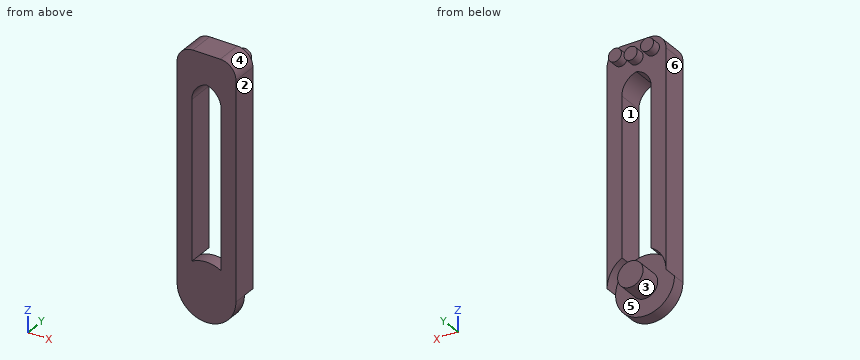
from build123d import *

# Parameters (mm, degrees)
F1_DEPTH    = 1.27
F3_R        = 1.524
F5_T1_DEPTH = 1.27
F2_R        = 1.2397519619
F6_DEPTH    = 2.1971
F4_R        = 0.6356353333
F4_R_2      = 0.6409754112
F7_DEPTH    = 3.429
F9_DEPTH    = 2.54


# Not quite as in the source:
# - a fillet or chamfer that OpenCascade refuses, or shapes differently, is made with other operations: its cross-section is extruded or revolved along the edge and cut away or added


with BuildPart() as f1:
    # F0 (on Front) → F1 (new body)
    with BuildSketch(Plane.XZ):
        with BuildLine():
            ThreePointArc((1.4341250062, 5.3522273875), (2.4839773751, 4.3023750186), (2.8682500124, 2.8682500124))
            Line((2.8682500124, 2.8682500124), (2.8682500124, 25.4276227206))
            Line((2.8682500124, 25.4276227206), (0, 25.4276227206))
            Line((0, 25.4276227206), (-1.4341250062, 25.4276227206))
            Line((-1.4341250062, 25.4276227206), (-2.8682500124, 25.4276227206))
            Line((-2.8682500124, 25.4276227206), (-2.8682500124, 2.8682500124))
            ThreePointArc((-2.8682500124, 2.8682500124), (-2.4839773751, 4.3023750186), (-1.4341250062, 5.3522273875))
            Line((-1.4341250062, 5.3522273875), (-1.4341250062, 22.6080268621))
            Line((-1.4341250062, 22.6080268621), (1.4341250062, 22.6080268621))
            Line((1.4341250062, 22.6080268621), (1.4341250062, 5.3522273875))
        make_face()
        with BuildLine():
            ThreePointArc((-2.8682500124, 2.8682500124), (0, 0), (2.8682500124, 2.8682500124))
            ThreePointArc((2.8682500124, 2.8682500124), (2.4839773751, 4.3023750186), (1.4341250062, 5.3522273875))
            ThreePointArc((1.4341250062, 5.3522273875), (0, 5.7365000248), (-1.4341250062, 5.3522273875))
            ThreePointArc((-1.4341250062, 5.3522273875), (-2.4839773751, 4.3023750186), (-2.8682500124, 2.8682500124))
        make_face()
    extrude(amount=F1_DEPTH)

    # F3
    f3_edges = [f1.edges().sort_by_distance(p)[0] for p in [
        (2.86825, -0.635, 25.427623),
        (-2.86825, -0.635, 25.427623),
    ]]
    fillet(f3_edges, radius=F3_R)

    # F5: fillet of radius 1.905 on 2 edges, made by hand

    # F5_s2 → F5_t1 (join)
    with BuildSketch(Plane.XZ):
        with BuildLine():
            ThreePointArc((-0.4708749938, 22.6080268621), (0.8761634244, 22.0500652803), (1.4341250062, 20.7030268621))
            Line((1.4341250062, 20.7030268621), (1.4341250062, 22.6080268621))
            Line((1.4341250062, 22.6080268621), (-0.4708749938, 22.6080268621))
        make_face()
        with BuildLine():
            ThreePointArc((-1.4341250062, 20.7030268621), (-0.8761634244, 22.0500652803), (0.4708749938, 22.6080268621))
            Line((0.4708749938, 22.6080268621), (-1.4341250062, 22.6080268621))
            Line((-1.4341250062, 22.6080268621), (-1.4341250062, 20.7030268621))
        make_face()
    extrude(amount=F5_T1_DEPTH)

    # F2 (on face) → F6 (join)
    with BuildSketch(Plane(origin=(0, 0, 0), x_dir=(-1, 0, 0), z_dir=(0, 1, 0))):
        with Locations((0, 2.8682500124)):
            Circle(F2_R)
    extrude(amount=F6_DEPTH)

    # F4 (on face) → F7 (join)
    with BuildSketch(Plane.XZ.offset(1.27)):
        with Locations((-1.5970880988, 24.1730304042)):
            Circle(F4_R)
        with Locations((1.5335635452, 24.1730304042)):
            Circle(F4_R)
        with Locations((0, 23.8491314396)):
            Circle(F4_R_2)
    extrude(amount=-F7_DEPTH)

    # F8 (on face) → F9 (join)
    with BuildSketch(Plane.XZ.offset(1.27)):
        with BuildLine():
            ThreePointArc((1.4341250062, 5.3522273875), (2.4839773751, 4.3023750186), (2.8682500124, 2.8682500124))
            Line((2.8682500124, 2.8682500124), (2.8682500124, 23.9036227206))
            ThreePointArc((2.8682500124, 23.9036227206), (1.7143439066, 22.42524303), (0, 23.1855921473))
            ThreePointArc((0, 23.1855921473), (-1.7143439066, 22.42524303), (-2.8682500124, 23.9036227206))
            Line((-2.8682500124, 23.9036227206), (-2.8682500124, 22.548914654))
            Line((-2.8682500124, 22.548914654), (-2.8682500124, 2.8682500124))
            ThreePointArc((-2.8682500124, 2.8682500124), (-2.4839773751, 4.3023750186), (-1.4341250062, 5.3522273875))
            Line((-1.4341250062, 5.3522273875), (-1.4341250062, 20.7030268621))
            ThreePointArc((-1.4341250062, 20.7030268621), (-1.0334590554, 21.8717886293), (0, 22.548914654))
            ThreePointArc((0, 22.548914654), (1.0334590554, 21.8717886293), (1.4341250062, 20.7030268621))
            Line((1.4341250062, 20.7030268621), (1.4341250062, 5.3522273875))
        make_face()
        with BuildLine():
            ThreePointArc((-2.8682500124, 23.9036227206), (-1.7143439066, 22.42524303), (0, 23.1855921473))
            ThreePointArc((0, 23.1855921473), (-0.1797499876, 23.9036227206), (0, 24.6216532939))
            ThreePointArc((0, 24.6216532939), (-0.5605736103, 25.2106909273), (-1.3442500124, 25.4276227206))
            ThreePointArc((-1.3442500124, 25.4276227206), (-2.4218807469, 24.9812534551), (-2.8682500124, 23.9036227206))
        make_face()
        with BuildLine():
            ThreePointArc((0, 23.1855921473), (1.7143439066, 22.42524303), (2.8682500124, 23.9036227206))
            ThreePointArc((2.8682500124, 23.9036227206), (2.4218807469, 24.9812534551), (1.3442500124, 25.4276227206))
            ThreePointArc((1.3442500124, 25.4276227206), (0.5605736103, 25.2106909273), (0, 24.6216532939))
            ThreePointArc((0, 24.6216532939), (0.1341296782, 24.2737166148), (0.1797499876, 23.9036227206))
            ThreePointArc((0.1797499876, 23.9036227206), (0.1341296782, 23.5335288264), (0, 23.1855921473))
        make_face()
        with BuildLine():
            ThreePointArc((0, 24.6216532939), (-0.1797499876, 23.9036227206), (0, 23.1855921473))
            ThreePointArc((0, 23.1855921473), (0.1341296782, 23.5335288264), (0.1797499876, 23.9036227206))
            ThreePointArc((0.1797499876, 23.9036227206), (0.1341296782, 24.2737166148), (0, 24.6216532939))
        make_face()
        with BuildLine():
            ThreePointArc((0, 24.6216532939), (0.5605736103, 25.2106909273), (1.3442500124, 25.4276227206))
            Line((1.3442500124, 25.4276227206), (-1.3442500124, 25.4276227206))
            ThreePointArc((-1.3442500124, 25.4276227206), (-0.5605736103, 25.2106909273), (0, 24.6216532939))
        make_face()
    extrude(amount=-F9_DEPTH)


solid = f1.part
Part model, mm, in its own coordinate system. Face numbers are marked on the shaded views. A direction names the side the tool comes from. Coordinates: 2 decimals unless noted, no trailing zeros. Loops run counter-clockwise (first coordinate to the right, second up) from the corner with the lowest first, then second, coordinate; pieces in that order, holes last. Notation, with made-up numbers: M 8.5,-13.5 L 48.5,-13.5 A29 cw 48.5,6.5 Z; hole C -39,-38 d10. An arc over 180 degrees is marked long. Use a Markdown table: item, result. Add a question column.
Q1. Mould opens along Z. For the marked faces 4, 5 and 6 say: +Z half, -Z half, draft (parallel to the pull), parting line (faces both ways), or undercut.
Q2. Cut at D-D (x = 2.45). Write the cut outline in (y, z), and give its area (3 significant figures).
Q3. Cut at C-C (y = -0.6). Write the cut outline in (x, z) (1 decimal), and give its area (3 significant figures).
Q4. Probe L1, parallel to X at y = 0.9, z = 15; L2, parallel to Z at x = 0, y = 1.4; L3, parallel to Y at x = 2.3, z = 5.25. List the from-to ranges inside material, lowest first.
Q5. Cut at A-A (z = 9). Write the cut outline in (x, y).
Q6. Pin check, flat tips, straight feed: P1, Ø1, axis at x = 1, z = 14, coming from the +Y side; P2, Ø1, axis at x = 1.5, z = 24.5, coming from the +Y side; P3, Ø2, axis at x = -1.5, y = -0.5, coming from the -Z side; P4, Ø1.5, axis at x = 0, z = 15.5, coming from the -Y side. Stop position of each tip, or through.
Q7. Which spindle directions (+Z, -Z, +X, -X, +Y, -Y) get a long thin tool onto all of the face, cutting with end or side? Do the marked faces 1, 2 and 3. Say none if no direction does.
Q8. Cut at B-B (y = 0.65). Write the cut outline in (x, z) (1 decimal).
Worked out:
| question | item | result |
|---|---|---|
| 1 | face 4 | +Z half |
| 1 | face 5 | undercut |
| 1 | face 6 | draft |
| 2 | outline | M -1.27,1.38 L 0,1.38 L 0,4.36 L 1.27,4.36 L 1.27,24.95 L -1.27,24.95 Z |
| 2 | area | 56.1 mm2 |
| 3 | outline | M -2.9,2.9 A2.9 ccw 2.9,2.9 L 2.9,23.9 A1.5 ccw 1.3,25.4 L -1.3,25.4 A1.5 ccw -2.9,23.9 Z; hole M -1.4,5.4 A2.9 cw 1.4,5.4 L 1.4,20.7 A1.9 ccw 0,22.5 A1.9 ccw -1.4,20.7 Z |
| 3 | area | 94.1 mm2 |
| 4 | L1 | x = -2.87 to -1.43, 1.43 to 2.87 |
| 4 | L2 | z = 1.63 to 4.11, 23.21 to 24.49 |
| 4 | L3 | y = -1.27 to 1.27 |
| 5 | outline | M -2.87,-1.27 L -1.43,-1.27 L -1.43,1.27 L -2.87,1.27 Z; M 1.43,-1.27 L 2.87,-1.27 L 2.87,1.27 L 1.43,1.27 Z |
| 6 | P1 | stops at y = 1.27 |
| 6 | P2 | stops at y = 2.16 |
| 6 | P3 | stops at z = 0.04 |
| 6 | P4 | passes through |
| 7 | face 1 | +Y, -Y |
| 7 | face 2 | +Z, -Z, +X, +Y, -Y |
| 7 | face 3 | +Y |
| 8 | outline | M -2.9,2.9 A2.9 cw -1.4,5.4 L -1.4,20.7 A1.9 cw 0,22.5 A1.9 cw 1.4,20.7 L 1.4,5.4 A2.9 cw 2.9,2.9 L 2.9,23.9 A1.5 ccw 1.3,25.4 L -1.3,25.4 A1.5 ccw -2.9,23.9 Z; C 0,2.9 d2.5 |
